from build123d import *

# Parameters (mm, degrees)
BOSS_EXTRUDE1_DEPTH       = 6.35
F_4_CLEARANCE_HOLE1_D     = 3.2639
F_4_CLEARANCE_HOLE1_DEPTH = 9.652
F_4_CLEARANCE_HOLE1_TIP   = 0.980574487
FILLET1_R                 = 12.7


with BuildPart() as part:
    # Sketch1 → Boss-Extrude1 (new body)
    with BuildSketch(Plane.XY):
        Polygon((0.838479943, 39.56529588), (-30.911520057, -15.42731726), (32.588479943, -15.42731726), align=None)
    extrude(amount=BOSS_EXTRUDE1_DEPTH)

    # #4 Clearance Hole1
    with Locations(Plane(origin=(-12.712258743, 3.394727996, 6.35), x_dir=(1, 0, 0), z_dir=(0, 0, 1))):
        with Locations((0, 0), (27.101477372, 0)):
            Hole(F_4_CLEARANCE_HOLE1_D / 2, depth=F_4_CLEARANCE_HOLE1_DEPTH)
            with Locations((0, 0, -(F_4_CLEARANCE_HOLE1_DEPTH + F_4_CLEARANCE_HOLE1_TIP / 2))):  # 118° drill point
                Cone(0, F_4_CLEARANCE_HOLE1_D / 2, F_4_CLEARANCE_HOLE1_TIP, mode=Mode.SUBTRACT)

    # Fillet1
    fillet1_edges = [part.edges().sort_by_distance(p)[0] for p in [
        (32.588479943, -15.42731726, 3.175),
        (-30.911520057, -15.42731726, 3.175),
        (0.838479943, 39.56529588, 3.175),
    ]]
    fillet(fillet1_edges, radius=FILLET1_R)


solid = part.part
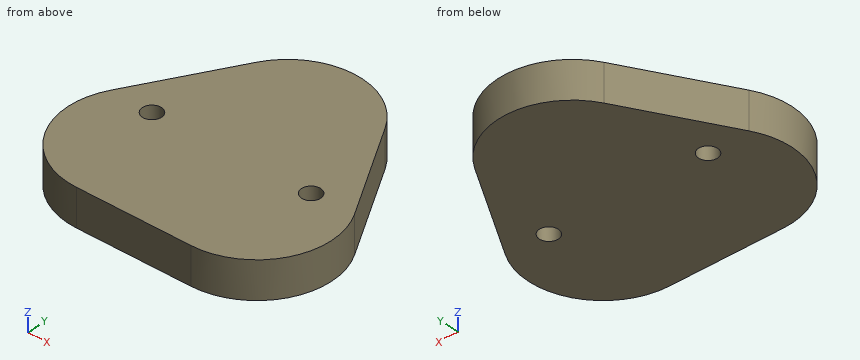
Can you work these out from the model? Positions are in its coordinate system, mm. Give positions to 0.01 mm unless a question says otherwise; leave off trailing zeros. Loops run counter-clockwise (first coordinate to the right, second up) from the corner with the lowest first, then second, coordinate; pieces in that order, holes last. Notation, with made-up numbers: M 23.5,83 L 64.5,83 A27 ccw 64.5,105 Z; hole C -39,29 d8. An arc over 180 degrees is marked long. One line per item, written item: value.
1) Imagine slicing it at B-B on z = 2.5. Write out the boundary of the cut face in (x, y), and give its area (3 significant figures).
Geometry check:
outline: M -19.91,3.62 A12.7 ccw -8.91,-15.43 L 10.59,-15.43 A12.7 ccw 21.59,3.62 L 11.84,20.52 A12.7 ccw -10.16,20.52 Z; hole C -12.71,3.39 d3.26; hole C 14.39,3.39 d3.26
area: 1,400 mm²
2) Imagine slicing it at A-A on x = 13.5. Write out the boundary of the cut face in (y, z), and give its area (3 significant figures).
Geometry check:
outline: M -15.09,0 L 2.03,0 L 2.03,6.35 L -15.09,6.35 Z; M 4.76,0 L 17.63,0 L 17.63,6.35 L 4.76,6.35 Z
area: 190 mm²
3) Imagine slicing it at C-C on y = 17. Write out the boundary of the cut face in (x, z).
Geometry check:
outline: M -12.19,0 L 13.87,0 L 13.87,6.35 L -12.19,6.35 Z
4) Imagine slicing it at D-D on x = -7.5. Write out the boundary of the cut face in (y, z), and give its area (3 significant figures).
Geometry check:
outline: M -15.43,0 L 23.74,0 L 23.74,6.35 L -15.43,6.35 Z
area: 249 mm²
5) Please list where these lines run through material, in increasing order: line 1 (X direction, y = 2, z = 3.25); line 2 (Y direction, x = -12, z = 3); line 3 (Y direction, x = -12.5, z = 4).
Geometry check:
line 1: x = -20.7 to -13.56, -11.86 to 13.54, 15.24 to 22.38
line 2: y = -15.05 to 1.93, 4.86 to 17.33
line 3: y = -14.91 to 1.78, 5.01 to 16.46
6) I'm going to push flat-ended pins straight in: pin 1 (2 mm diameter, centred on y = 4, z = 2.5, fed in from +X); pin 2 (4 mm diameter, centred on x = 14.39, y = 3.39, fed in from +Z); pin 3 (1 mm diameter, centred on y = 21, z = 3.5, fed in from +X); pin 4 (1.5 mm diameter, centred on x = 16, y = 18, fed in from -Z). Where does each tip first touch, or does it pass through?
Geometry check:
pin 1: stops at x = 21.93
pin 2: stops at z = 6.35
pin 3: stops at x = 11.85
pin 4: passes through
